from build123d import *

# Parameters (mm, degrees)
F1_DEPTH = 25.4
F2_R     = 1
F3_R     = 1


with BuildPart() as f1:
    # F0 (on Top) → F1 (new body)
    with BuildSketch(Plane.XY):
        Polygon((-8.5, 0), (0, 0), (0, 1), (-9.5, 1), (-9.5, -6), (-6, -6), (-6, -5), (-8.5, -5), align=None)
        Polygon((0, 1), (0, 0), (8.5, 0), (8.5, -5), (6, -5), (6, -6), (9.5, -6), (9.5, 1), align=None)
    extrude(amount=F1_DEPTH)

    # F2
    f2_edges = [f1.edges().sort_by_distance(p)[0] for p in [
        (-9.5, 1, 12.7),
        (9.5, 1, 12.7),
    ]]
    fillet(f2_edges, radius=F2_R)

    # F3
    f3_edges = [f1.edges().sort_by_distance(p)[0] for p in [
        (-9.5, -6, 12.7),
        (9.5, -6, 12.7),
    ]]
    fillet(f3_edges, radius=F3_R)


solid = f1.part
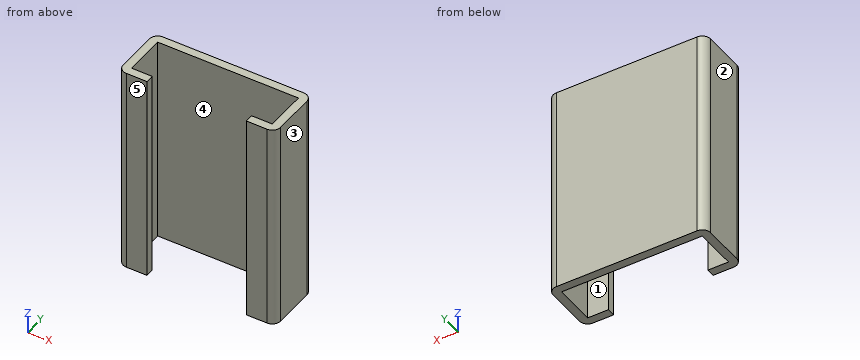
Check sheet for the modelled part. Datum: model origin and axes. Units: mm. Face numbers are marked on the shaded views. A direction names the side the tool comes from. Give positions to 0.01 mm unless a question says otherwise; leave off trailing zeros. Write each loop counter-clockwise with the first axis right and the second up, starting at its lowest first coordinate (ties: lowest second). Pieces come first, ordered by that corner, then holes. Notation, with made-up numbers: (-18.75, -37.75) -> (1.25, -37.75) arc R12 cw to (1.25, -20.75) -> close; hole circle Ø5 at (8.25, 57.25). An arc over 180 degrees is marked (long way). Use one line per item in the form item = value. Start each with the question number.
1. Section check D-D (x = 1). Record the cut outline in (y, z), and give its area (3 significant figures).
2. Access from +Z, -Z, +X, -X, +Y, -Y to the whole of each face (thin tool, end or side, straight path). Record for the marked faces 1 and 2.
3. Thickness scan on line 1 along X through (y, z) = (-1, 19.25); line 2 along Y through (x, z) = (-6.5, 9.5); line 3 along Y through (x, z) = (-4, 13.5). Record the ranges inside material, lowest first. Write a range as from..to.
4. Mould release check, pull along Y, two halves, no side actions. Record for the marked faces 3, 4 and 5: pulls with the +Y half, pulls with the -Y half, needs draft (parallel to the pull), parting line crosses it, or undercut.
5. Section check A-A (x = -7.25). Record the cut outline in (y, z).
6. Section check C-C (z = 10.5). Record the cut outline in (x, y).
7. Go/stop test with flat-tipped pins: P1, Ø4, axis at x = -1, y = -0.5, coming from the -Z side; P2, Ø1, axis at x = 0, z = 18, coming from the -Y side. Record where each tip stops, or that it passes through.
8. Section check B-B (y = -1.25). Record the cut outline in (x, z).
Conclusion:
q1.outline = (0, 0) -> (1, 0) -> (1, 25.4) -> (0, 25.4) -> close
q1.area = 25.4 mm²
q2.face_1 = +Z, -Z
q2.face_2 = +Z, -Z, -X, +Y, -Y
q3.line_1 = -9.5..-8.5, 8.5..9.5
q3.line_2 = -6..-5, 0..1
q3.line_3 = 0..1
q4.face_3 = needs draft
q4.face_4 = undercut
q4.face_5 = pulls with the -Y half
q5.outline = (-6, 0) -> (-5, 0) -> (-5, 25.4) -> (-6, 25.4) -> close; (0, 0) -> (1, 0) -> (1, 25.4) -> (0, 25.4) -> close
q6.outline = (-9.5, -5) arc R1 ccw to (-8.5, -6) -> (-6, -6) -> (-6, -5) -> (-8.5, -5) -> (-8.5, 0) -> (8.5, 0) -> (8.5, -5) -> (6, -5) -> (6, -6) -> (8.5, -6) arc R1 ccw to (9.5, -5) -> (9.5, 0) arc R1 ccw to (8.5, 1) -> (-8.5, 1) arc R1 ccw to (-9.5, 0) -> close
q7.P1 = 0
q7.P2 = 0
q8.outline = (-9.5, 0) -> (-8.5, 0) -> (-8.5, 25.4) -> (-9.5, 25.4) -> close; (8.5, 0) -> (9.5, 0) -> (9.5, 25.4) -> (8.5, 25.4) -> close
